Here's how the part is built. I have some questions about the finished solid (model axes, mm). Face numbers are marked on the shaded views. A direction names the side the tool comes from. Round coordinates to 2 decimals unless told otherwise and drop trailing zeros. Write each loop counter-clockwise with the first axis right and the second up, starting at its lowest first coordinate (ties: lowest second). Pieces come first, ordered by that corner, then holes. Notation, with made-up numbers: (32, 70.25) -> (54, 70.25) arc R15 cw to (54, 96.25) -> close; hole circle Ø3 at (69, 36.5). An arc over 180 degrees is marked (long way). Answer in a Markdown table with one row per item. Add a question column.
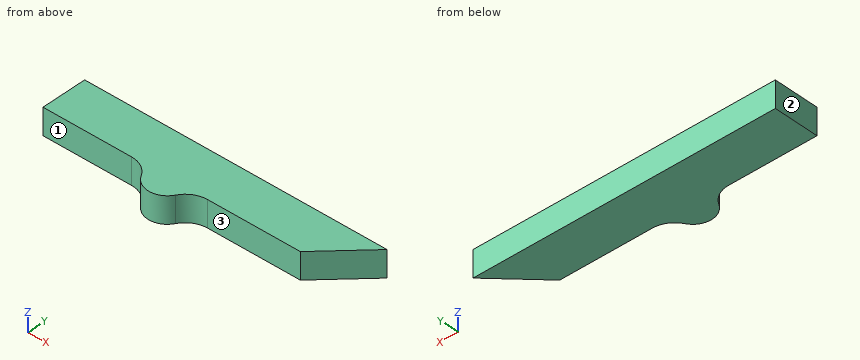
from build123d import *

# Parameters (mm, degrees)
BOSS_EXTRUDE1_DEPTH = 1.2


with BuildPart() as part:
    # Sketch1 → Boss-Extrude1 (new body)
    with BuildSketch(Plane.XY):
        with BuildLine():
            Line((23.337922061, 10.61), (25.387922061, 12.66))
            Line((25.387922061, 12.66), (11.625, 12.66))
            Line((11.625, 12.66), (11.625, 10.61))
            Line((11.625, 10.61), (15.649410223, 10.61))
            ThreePointArc((15.649410223, 10.61), (16.199410223, 10.462627944), (16.602038167, 10.06))
            ThreePointArc((16.602038167, 10.06), (17.381461031, 9.61), (18.160883894, 10.06))
            ThreePointArc((18.160883894, 10.06), (18.563511838, 10.462627944), (19.113511838, 10.61))
            Line((19.113511838, 10.61), (23.337922061, 10.61))
        make_face()
    extrude(amount=BOSS_EXTRUDE1_DEPTH)


solid = part.part
Item 1: For P1, Ø1.5, axis at x = 21, y = 10.5, coming from the +Z side, with a flat end and sliding along its axis, tell me the tip position at first contact or that it passes through.
Item 2: If we section it at A-A on z = 0.6: Please give me the cut outline in (x, y) (3 decimals), then the cut area to 3 significant figures.
Item 3: On a 3-axis mill with a long thin cutter (end or side, diameter ignored), from which of +Z, -Z, +X, -X, +Y, -Y can I reach the whole of each face in a straight line? I mean the marked faces 1, 2 and 3. Say none if no direction works.
Item 4: I need wall thicknesses on line 1 along Y through (x, z) = (15.5, 0.4); line 2 along Y through (x, z) = (16.25, 0.8); line 3 along X through (y, z) = (11.6, 1) (3 decimals). Which ranges of each line are inside material? Lowest first, please. Write a range as from..to.
Item 5: If we section it at C-C on y = 9.9: Please give me the cut outline in (x, z).
Item 6: If we section it at B-B on x = 21.75: Please give me the cut outline in (y, z), then the cut area to 3 significant figures.
Results list:
| question | item | result |
|---|---|---|
| 1 | P1 | z = 1.2 |
| 2 | outline | (11.625, 10.61) -> (15.649, 10.61) arc R1.1 cw to (16.602, 10.06) arc R0.9 ccw to (18.161, 10.06) arc R1.1 cw to (19.114, 10.61) -> (23.338, 10.61) -> (25.388, 12.66) -> (11.625, 12.66) -> close |
| 2 | area | 27.8 mm² |
| 3 | face 1 | +Z, -Z, -X, -Y |
| 3 | face 2 | +Z, -Z, -X, +Y, -Y |
| 3 | face 3 | +Z, -Z, +X, -Y |
| 4 | line 1 | 10.61..12.66 |
| 4 | line 2 | 10.43..12.66 |
| 4 | line 3 | 11.625..24.328 |
| 5 | outline | (16.72, 0) -> (18.04, 0) -> (18.04, 1.2) -> (16.72, 1.2) -> close |
| 6 | outline | (10.61, 0) -> (12.66, 0) -> (12.66, 1.2) -> (10.61, 1.2) -> close |
| 6 | area | 2.46 mm² |
